Read the model definition and answer for the solid it produces. Units are mm, in the model's axes. A direction names the side the tool comes from. Round coordinates to 2 decimals unless told otherwise and drop trailing zeros.
from build123d import *

# Parameters (mm, degrees)
SKETCH1_W                                  = 128
SKETCH1_H                                  = 105
BOSS_EXTRUDE1_DEPTH                        = 3
SKETCH2_W                                  = 13.5
SKETCH2_H                                  = 105
BOSS_EXTRUDE2_DEPTH                        = 2.9
BOSS_EXTRUDE9_DEPTH                        = 7
FILLET1_R                                  = 6
FILLET2_R                                  = 1
CUT_EXTRUDE1_DEPTH                         = 7
SKETCH3_W                                  = 3
SKETCH3_H                                  = 95
BOSS_EXTRUDE10_DEPTH                       = 20
SKETCH11_R                                 = 1
CUT_EXTRUDE2_DEPTH                         = 20
SKETCH13_R                                 = 1
CUT_EXTRUDE3_DEPTH                         = 20
MIRROR1_AT_THE_SECOND_PLANE_COPY_1_SKETC_R = 1
MIRROR1_AT_THE_SECOND_PLANE_COPY_1_DEPTH   = 20
SKETCH4_W                                  = 50
SKETCH4_H                                  = 3
SKETCH4_W_2                                = 25
BOSS_EXTRUDE11_DEPTH                       = 20
CUT_EXTRUDE4_REACH                         = 140.569
SKETCH14_W                                 = 40
SKETCH14_H                                 = 10
SKETCH15_W                                 = 50
SKETCH15_H                                 = 15
BOSS_EXTRUDE12_DEPTH                       = 1.5
SKETCH17_R                                 = 1
CUT_EXTRUDE5_DEPTH                         = 1.5
SKETCH18_W                                 = 12
SKETCH18_H                                 = 95
SKETCH18_R                                 = 1
BOSS_EXTRUDE13_DEPTH                       = 1.5


with BuildPart() as part:
    # Sketch1 → Boss-Extrude1 (new body)
    with BuildSketch(Plane(origin=(0, 0, 0), x_dir=(1, 0, 0), z_dir=(0, 1, 0))):
        Rectangle(SKETCH1_W, SKETCH1_H)
    extrude(amount=BOSS_EXTRUDE1_DEPTH)

    # Sketch2 → Boss-Extrude2 (add)
    with BuildSketch(Plane(origin=(0, 0, 0), x_dir=(1, 0, 0), z_dir=(0, 1, 0))):
        with Locations((-70.75, 0)):
            Rectangle(SKETCH2_W, SKETCH2_H)
        with Locations((70.75, 0)):
            Rectangle(SKETCH2_W, SKETCH2_H)
    extrude(amount=BOSS_EXTRUDE2_DEPTH)

    # Sketch5 → Boss-Extrude9 (add)
    with BuildSketch(Plane(origin=(0, 3, 0), x_dir=(1, 0, 0), z_dir=(0, 1, 0))):
        Polygon((-6.5, -19), (-6.5, -17.5), (-13, -17.5), (-13, 17.5), (13, 17.5), (13, -17.5), (6.5, -17.5), (6.5, -19), (14.5, -19), (14.5, 19), (-14.5, 19), (-14.5, -19), align=None)
    extrude(amount=BOSS_EXTRUDE9_DEPTH)

    # Fillet1
    fillet1_edges = [part.edges().sort_by_distance(p)[0] for p in [
        (-6.5, 10, 18.25),
        (6.5, 10, 18.25),
    ]]
    fillet(fillet1_edges, radius=FILLET1_R)

    # Fillet2
    fillet2_edges = [part.edges().sort_by_distance(p)[0] for p in [
        (-13, 6.5, 17.5),
        (13, 6.5, 17.5),
        (-13, 6.5, -17.5),
        (14.5, 6.5, -19),
        (14.5, 6.5, 19),
        (13, 6.5, -17.5),
        (-14.5, 6.5, -19),
        (-14.5, 6.5, 19),
    ]]
    fillet(fillet2_edges, radius=FILLET2_R)

    # Sketch10 → Cut-Extrude1 (cut)
    with BuildSketch(Plane(origin=(0, 3, 0), x_dir=(1, 0, 0), z_dir=(0, 1, 0))):
        Polygon((-54, 36.137163962), (-54, 6), (-15.708074024, 6), align=None)
        with BuildLine():
            Line((-6, 42.5), (-45.915455387, 42.5))
            Line((-45.915455387, 42.5), (-14.5, 17.774873075))
            Line((-14.5, 17.774873075), (-14.5, 18))
            ThreePointArc((-14.5, 18), (-14.207106781, 18.707106781), (-13.5, 19))
            Line((-13.5, 19), (-6, 19))
            Line((-6, 19), (-6, 42.5))
        make_face()
        with BuildLine():
            Line((45.915455387, 42.5), (6, 42.5))
            Line((6, 42.5), (6, 19))
            Line((6, 19), (13.5, 19))
            ThreePointArc((13.5, 19), (14.207106781, 18.707106781), (14.5, 18))
            Line((14.5, 18), (14.5, 17.774873075))
            Line((14.5, 17.774873075), (45.915455387, 42.5))
        make_face()
        Polygon((15.708074024, 6), (54, 6), (54, 36.137163962), align=None)
        Polygon((15.708074024, -6), (54, -36.137163962), (54, -6), align=None)
        with BuildLine():
            Line((6, -19), (6, -42.5))
            Line((6, -42.5), (45.915455387, -42.5))
            Line((45.915455387, -42.5), (14.5, -17.774873075))
            Line((14.5, -17.774873075), (14.5, -18))
            ThreePointArc((14.5, -18), (14.207106781, -18.707106781), (13.5, -19))
            Line((13.5, -19), (6.5, -19))
            Line((6.5, -19), (6, -19))
        make_face()
        with BuildLine():
            Line((-14.5, -17.774873075), (-45.915455387, -42.5))
            Line((-45.915455387, -42.5), (-6, -42.5))
            Line((-6, -42.5), (-6, -19))
            Line((-6, -19), (-6.5, -19))
            Line((-6.5, -19), (-13.5, -19))
            ThreePointArc((-13.5, -19), (-14.207106781, -18.707106781), (-14.5, -18))
            Line((-14.5, -18), (-14.5, -17.774873075))
        make_face()
        Polygon((-54, -6), (-54, -36.137163962), (-15.708074024, -6), align=None)
    extrude(amount=-CUT_EXTRUDE1_DEPTH, mode=Mode.SUBTRACT)

    # Sketch3 → Boss-Extrude10 (add)
    with BuildSketch(Plane(origin=(0, 0, 0), x_dir=(1, 0, 0), z_dir=(0, 1, 0))):
        with Locations((-79, 0)):
            Rectangle(SKETCH3_W, SKETCH3_H)
        with Locations((79, 0)):
            Rectangle(SKETCH3_W, SKETCH3_H)
    extrude(amount=BOSS_EXTRUDE10_DEPTH)

    # Sketch11 → Cut-Extrude2 (cut)
    with BuildSketch(Plane(origin=(0, 3, 0), x_dir=(1, 0, 0), z_dir=(0, 1, 0))):
        with Locations(Location((-63.3, -41, 0), (0, 0, 270))):
            Circle(SKETCH11_R)
        with Locations(Location((-63.3, -34.5, 0), (0, 0, 270))):
            Circle(SKETCH11_R)
        with Locations(Location((-63.3, 34.5, 0), (0, 0, 270))):
            Circle(SKETCH11_R)
        with Locations(Location((-63.3, 41, 0), (0, 0, 270))):
            Circle(SKETCH11_R)
        with Locations(Location((63.3, 41, 0), (0, 0, 270))):
            Circle(SKETCH11_R)
        with Locations(Location((63.3, 34.5, 0), (0, 0, 270))):
            Circle(SKETCH11_R)
        with Locations(Location((63.3, -34.5, 0), (0, 0, 270))):
            Circle(SKETCH11_R)
        with Locations(Location((63.3, -41, 0), (0, 0, 270))):
            Circle(SKETCH11_R)
    extrude(amount=-CUT_EXTRUDE2_DEPTH, mode=Mode.SUBTRACT)

    # Sketch13 → Cut-Extrude3 (cut)
    with BuildSketch(Plane(origin=(-77.5, 0, 0), x_dir=(0, 0, -1), z_dir=(1, 0, 0))):
        with Locations((-41, 14.842473729)):
            Circle(SKETCH13_R)
        with Locations((-34.5, 14.842473729)):
            Circle(SKETCH13_R)
    cut_extrude3 = extrude(amount=-CUT_EXTRUDE3_DEPTH, mode=Mode.SUBTRACT)

    # Mirror1: Cut-Extrude3 across plane
    add(cut_extrude3.mirror(Plane.XY), mode=Mode.SUBTRACT)

    # Mirror1 at the second plane: Cut-Extrude3 across plane
    add(cut_extrude3.mirror(Plane(origin=(0, 0, 0), x_dir=(0, 0, 1), z_dir=(1, 0, 0))), mode=Mode.SUBTRACT)

    # Mirror1 at the second plane copy 1 sketc → Mirror1 at the second plane copy 1 (cut)
    with BuildSketch(Plane.ZY.offset(-77.5)):
        with Locations((-41, 14.842473729)):
            Circle(MIRROR1_AT_THE_SECOND_PLANE_COPY_1_SKETC_R)
        with Locations((-34.5, 14.842473729)):
            Circle(MIRROR1_AT_THE_SECOND_PLANE_COPY_1_SKETC_R)
    extrude(amount=-MIRROR1_AT_THE_SECOND_PLANE_COPY_1_DEPTH, mode=Mode.SUBTRACT)

    # Sketch4 → Boss-Extrude11 (add)
    with BuildSketch(Plane(origin=(0, 0, 0), x_dir=(1, 0, 0), z_dir=(0, 1, 0))):
        with Locations((0, 54)):
            Rectangle(SKETCH4_W, SKETCH4_H)
        with Locations((-12.5, -54)):
            Rectangle(SKETCH4_W_2, SKETCH4_H)
        with Locations((12.5, -54)):
            Rectangle(SKETCH4_W_2, SKETCH4_H)
    extrude(amount=BOSS_EXTRUDE11_DEPTH)

    # Sketch14 → Cut-Extrude4 (cut, up to next)
    with BuildSketch(Plane.XY.offset(55.5), mode=Mode.PRIVATE) as cut_extrude4_sk1:
        with Locations((0, 10)):
            Rectangle(SKETCH14_W, SKETCH14_H)
    cut_extrude4_tool1 = extrude(cut_extrude4_sk1.sketch, amount=-CUT_EXTRUDE4_REACH, mode=Mode.PRIVATE) & part.part
    add(cut_extrude4_tool1.solids().sort_by_distance((0, 10, 55.5))[0], mode=Mode.SUBTRACT)

    # Sketch15 → Boss-Extrude12 (add)
    with BuildSketch(Plane(origin=(0, 20, 0), x_dir=(1, 0, 0), z_dir=(0, 1, 0))):
        with Locations((0, -48)):
            Rectangle(SKETCH15_W, SKETCH15_H)
    boss_extrude12 = extrude(amount=BOSS_EXTRUDE12_DEPTH)

    # Sketch17 → Cut-Extrude5 (cut)
    with BuildSketch(Plane(origin=(0, 21.5, 0), x_dir=(1, 0, 0), z_dir=(0, 1, 0))):
        with Locations(Location((18, -45.5, 0), (0, 0, 270))):
            Circle(SKETCH17_R)
        with Locations(Location((-18, -45.5, 0), (0, 0, 90))):
            Circle(SKETCH17_R)
    cut_extrude5 = extrude(amount=-CUT_EXTRUDE5_DEPTH, mode=Mode.SUBTRACT)

    # Mirror2: Boss-Extrude12, Cut-Extrude5 across plane
    add(boss_extrude12.mirror(Plane.XY))
    add(cut_extrude5.mirror(Plane.XY), mode=Mode.SUBTRACT)

    # Sketch18 → Boss-Extrude13 (add)
    with BuildSketch(Plane(origin=(0, 20, 0), x_dir=(1, 0, 0), z_dir=(0, 1, 0))):
        with Locations((-74.5, 0)):
            Rectangle(SKETCH18_W, SKETCH18_H)
        with Locations(Location((-72.5, -15, 0), (0, 0, 270))):
            Circle(SKETCH18_R, mode=Mode.SUBTRACT)
        with Locations(Location((-72.5, -7.5, 0), (0, 0, 270))):
            Circle(SKETCH18_R, mode=Mode.SUBTRACT)
        with Locations(Location((-72.5, 7.5, 0), (0, 0, 270))):
            Circle(SKETCH18_R, mode=Mode.SUBTRACT)
        with Locations(Location((-72.5, 15, 0), (0, 0, 270))):
            Circle(SKETCH18_R, mode=Mode.SUBTRACT)
    boss_extrude13 = extrude(amount=BOSS_EXTRUDE13_DEPTH)

    # Mirror3: Boss-Extrude13 across plane
    add(boss_extrude13.mirror(Plane(origin=(0, 0, 0), x_dir=(0, 0, 1), z_dir=(1, 0, 0))))


solid = part.part
Q1. Flat-ended cylindrical pins translate along their axes: pin 1 (3.5 mm diameter, centred on x = 41, y = 1.5, fed in from -Z); pin 2 (3.5 mm diameter, centred on x = -27, y = 1.5, fed in from +Z); pin 3 (1 mm diameter, centred on x = -64, z = -0.5, fed in from +Y). Find the tip coordinate at first contact, or state that the pin passes through.
Outcome:
pin 1: stops at z = -52.5
pin 2: stops at z = 52.5
pin 3: stops at y = 3
Q2. A cutting plane is placed at A-A, the plane z = -26. Give the number of separate pieces and of enclosed holes in the cut face, plus the area to 3 significant figures.
Outcome:
separate pieces: 5
enclosed holes: 0
area: 427 mm2
Q3. For a pull along X with two mould halves and no side action, classify faces 4 (the face through (-0.3, 15.4, 55.5)), 5 (the face through (-35.12, 1.52, 21.28)) as released by +X, released by -X, zero draft, split by the parting line, or undercut.
Outcome:
face 4: zero draft
face 5: undercut
Q4. For faces 1 (the face through (77.5, 11, 1)), 2 (the face through (20, 10, 54)), 3 (the face through (-34.59, 1.52, -20.86)), determine the directions among +Z, -Z, +X, -X, +Y, -Y from which every point of the face is accessible in a straight line to the end or side of a thin tool.
Outcome:
face 1: +Z, -Z
face 2: +Z
face 3: +Y, -Y
Q5. Straight lines are drawn through the part: probe 1 along Z at (x, y) = (-72.5, 20.6); probe 2 along X at (y, z) = (7.75, -8); probe 3 along X at (y, z) = (3.25, -25). For each, find the intervals that lie inside material, in ascending order.
Outcome:
probe 1: z = -47.5 to -16, -14 to -8.5, -6.5 to 6.5, 8.5 to 14, 16 to 47.5
probe 2: x = -80.5 to -77.5, -14.5 to -13, 13 to 14.5, 77.5 to 80.5
probe 3: x = -80.5 to -77.5, 77.5 to 80.5
